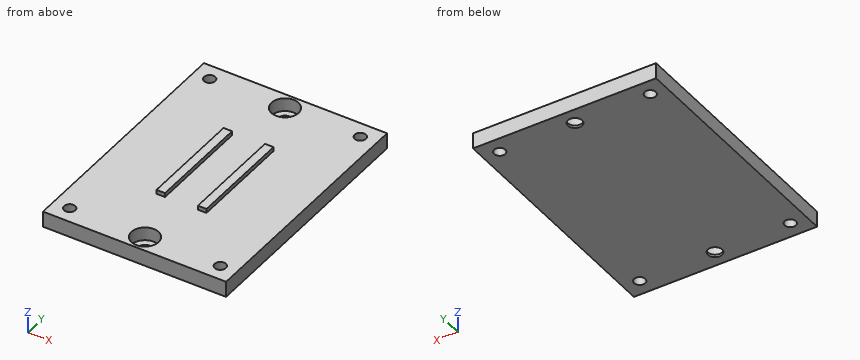
```python
from build123d import *

# Parameters (mm, degrees)
F0_W           = 44
F0_H           = 60
F1_DEPTH       = 3.8
F3_D           = 2.7
F4_D           = 3.4
F4_CBORE_D     = 6.5
F4_CBORE_DEPTH = 3.2
F5_W           = 2.05
F5_H           = 25
F6_DEPTH       = 1


with BuildPart() as f1:
    # F0 (on Top) → F1 (new body)
    with BuildSketch(Plane.XY):
        Rectangle(F0_W, F0_H)
    extrude(amount=F1_DEPTH)

    # F3 (through all)
    with Locations(Plane.XY.offset(3.8)):
        with Locations((-18.1, 26.1), (18.1, 26.1), (18.1, -26.1), (-18.1, -26.1)):
            Hole(F3_D / 2)

    # F4 (through all)
    with Locations(Plane.XY.offset(3.8)):
        with Locations((0, 26.1), (0, -26.1)):
            CounterBoreHole(F4_D / 2, F4_CBORE_D / 2, F4_CBORE_DEPTH)

    # F5 (on face) → F6 (join)
    with BuildSketch(Plane.XY.offset(3.8)):
        with Locations((-4.975, 0)):
            Rectangle(F5_W, F5_H)
        with Locations((4.975, 0)):
            Rectangle(F5_W, F5_H)
    extrude(amount=F6_DEPTH)


solid = f1.part
```
Model file for the job. Use its own axes, mm. Coordinates: 2 decimals unless noted, no trailing zeros. Write each loop counter-clockwise with the first axis right and the second up, starting at its lowest first coordinate (ties: lowest second). Pieces come first, ordered by that corner, then holes. Notation, with made-up numbers: (87.5, 12.25) - (126.5, 12.25) arc R20 ccw to (126.5, 20.25) - close; hole circle Ø1 at (13, 51). An arc over 180 degrees is marked (long way). One line per question, with ' | ' between items. Start each with the question number.
Q1. Cut at A-A, the plane x = 0. List the corners of the cut face in (y, z).
Q2. Cut at B-B, the plane z = 1.3. List the corners of the cut face in (x, y).
Q3. Pin check, flat tips, straight feed: pin 1 (5 mm diameter, centred on x = -1, y = 27, fed in from +Z); pin 2 (0.8 mm diameter, centred on x = 5, z = 4.5, fed in from -Y). Stop position of each tip, or through.
Q4. Drill centre lines: line 1 (Y direction, x = 0, z = 0.3); line 2 (Y direction, x = 0, z = 2); line 3 (X direction, y = -26.5, z = 0.55). Where is each one in solid material? Low to high. Write a range as [from, to].
Q5. Cut at C-C, the plane y = 26.1. List the corners of the cut face in (x, z).
Q6. Cut at D-D, the plane y = 1.5. List the corners of the cut face in (x, z).
Answer below:
1) outline: (-30, 0) - (-27.8, 0) - (-27.8, 0.6) - (-29.35, 0.6) - (-29.35, 3.8) - (-30, 3.8) - close; (-24.4, 0) - (24.4, 0) - (24.4, 0.6) - (22.85, 0.6) - (22.85, 3.8) - (-22.85, 3.8) - (-22.85, 0.6) - (-24.4, 0.6) - close; (27.8, 0) - (30, 0) - (30, 3.8) - (29.35, 3.8) - (29.35, 0.6) - (27.8, 0.6) - close
2) outline: (-22, -30) - (22, -30) - (22, 30) - (-22, 30) - close; hole circle Ø2.7 at (-18.1, -26.1); hole circle Ø2.7 at (-18.1, 26.1); hole circle Ø6.5 at (0, -26.1); hole circle Ø6.5 at (0, 26.1); hole circle Ø2.7 at (18.1, -26.1); hole circle Ø2.7 at (18.1, 26.1)
3) pin 1: z = 3.8 | pin 2: y = -12.5
4) line 1: [-30, -27.8], [-24.4, 24.4], [27.8, 30] | line 2: [-30, -29.35], [-22.85, 22.85], [29.35, 30] | line 3: [-22, -19.39], [-16.81, -1.65], [1.65, 16.81], [19.39, 22]
5) outline: (-22, 0) - (-19.45, 0) - (-19.45, 3.8) - (-22, 3.8) - close; (-16.75, 0) - (-1.7, 0) - (-1.7, 0.6) - (-3.25, 0.6) - (-3.25, 3.8) - (-16.75, 3.8) - close; (1.7, 0) - (16.75, 0) - (16.75, 3.8) - (3.25, 3.8) - (3.25, 0.6) - (1.7, 0.6) - close; (19.45, 0) - (22, 0) - (22, 3.8) - (19.45, 3.8) - close
6) outline: (-22, 0) - (22, 0) - (22, 3.8) - (6, 3.8) - (6, 4.8) - (3.95, 4.8) - (3.95, 3.8) - (-3.95, 3.8) - (-3.95, 4.8) - (-6, 4.8) - (-6, 3.8) - (-22, 3.8) - close
